from build123d import *

# Parameters (mm, degrees)
SKETCH1_R           = 34.671
BOSS_EXTRUDE1_DEPTH = 19.05
SKETCH5_R           = 5.08
CUT_EXTRUDE1_DEPTH  = 53.602841957
CHAMFER1_SIZE       = 6
CIRPATTERN1_COUNT   = 4
SKETCH8_R           = 3.3655
CUT_EXTRUDE2_DEPTH  = 53.602841957
CIRPATTERN2_COUNT   = 6


with BuildPart() as part:
    # Sketch1 → Boss-Extrude1 (new body)
    with BuildSketch(Plane(origin=(0, 0, 0), x_dir=(1, 0, 0), z_dir=(0, 1, 0))):
        with Locations(Location((0, 0, 0), (0, 0, 90))):
            Circle(SKETCH1_R)
    extrude(amount=BOSS_EXTRUDE1_DEPTH)

    # Sketch5 → Cut-Extrude1 (cut, through all)
    with BuildSketch(Plane.XZ):
        with Locations(Location((0, 0, 0), (0, 0, 270))):
            Circle(SKETCH5_R)
    extrude(amount=-CUT_EXTRUDE1_DEPTH, mode=Mode.SUBTRACT)

    # Chamfer1
    chamfer1_edges = [part.edges().sort_by_distance(p)[0] for p in [
        (0, 19.05, 5.08),
    ]]
    chamfer(chamfer1_edges, length=CHAMFER1_SIZE)

    # Sketch6 → #6-32 Tapped Hole1 (revolve, cut)
    with BuildSketch(Plane(origin=(0, 19.05, -13.5), x_dir=(0, 0, 1), z_dir=(1, 0, 0))):
        Polygon((0, 0), (0, 10.81269403), (1.35255, 10), (1.35255, 0), align=None)
    f_6_32_tapped_hole1 = revolve(axis=Axis((0, 25.4, -13.5), (0, -1, 0)), mode=Mode.SUBTRACT)

    # CirPattern1: #6-32 Tapped Hole1 ×4 about axis
    cirpattern1_axis = Axis((0, 0, 0), (0, 1, 0))
    for i in range(1, CIRPATTERN1_COUNT):
        add(f_6_32_tapped_hole1.rotate(cirpattern1_axis, i * 360 / CIRPATTERN1_COUNT), mode=Mode.SUBTRACT)

    # Sketch8 → Cut-Extrude2 (cut, through all)
    with BuildSketch(Plane(origin=(0, 19.05, 0), x_dir=(1, 0, 0), z_dir=(0, 1, 0))):
        with Locations(Location((0, 29.3624, 0), (0, 0, 270))):
            Circle(SKETCH8_R)
    cut_extrude2 = extrude(amount=-CUT_EXTRUDE2_DEPTH, mode=Mode.SUBTRACT)

    # CirPattern2: Cut-Extrude2 ×6 about axis
    cirpattern2_axis = Axis((0, 0, 0), (0, 1, 0))
    for i in range(1, CIRPATTERN2_COUNT):
        add(cut_extrude2.rotate(cirpattern2_axis, i * 360 / CIRPATTERN2_COUNT), mode=Mode.SUBTRACT)

    # Sketch9 → Cut-Revolve1 (revolve, cut)
    with BuildSketch(Plane.XY, mode=Mode.PRIVATE) as cut_revolve1_sk:
        Polygon((0, -2.570803014), (0, 0.5), (22.5, 0.5), (22.5, 0), (24.5, 0.5), (24.5, -7.98797561), (0, -7.98797561), align=None)
    cut_revolve1 = revolve(cut_revolve1_sk.sketch.rotate(Axis((0, -2.570803014, 0), (0, 1, 0)), 90), axis=Axis((0, -2.570803014, 0), (0, 1, 0)), mode=Mode.SUBTRACT)

    # Mirror1: Cut-Revolve1 across plane
    add(cut_revolve1.mirror(Plane(origin=(0, 9.525, 0), x_dir=(0, 0, 1), z_dir=(0, -1, 0))), mode=Mode.SUBTRACT)


solid = part.part
The model under review builds one solid part; all positions refer to its coordinate system, in mm. A direction names the side the tool comes from. Round coordinates to 2 decimals unless told otherwise and drop trailing zeros. Write each loop counter-clockwise with the first axis right and the second up, starting at its lowest first coordinate (ties: lowest second). Pieces come first, ordered by that corner, then holes. Notation, with made-up numbers: M -8,47 L 32,47 A3 ccw 32,51 Z; hole C 60.5,32 d10. An arc over 180 degrees is marked long. Answer as CSV lines item,"result". Start each with the question number.
Q1. Tool access review of faces 4 (the face through (-5.3, 0.5, -0.3)), 5 (the face through (10, 18.55, 5)), 6 (the face through (-23, 0, 10)): name each direction out of +Z, -Z, +X, -X, +Y, -Y from which nothing blocks a thin tool from reaching the whole face with its end or side.
Q2. Consider section B-B, the plane x = -26.5. Give the boundary of the cut face in (y, z), then the cut area to 3 significant figures.
Q3. Consider section A-A, the plane z = -29. Give the boundary of the cut face in (x, y).
Q4. Wall thickness on line 1 along Z through (x, y) = (26.5, 4); line 2 along X through (y, z) = (14, 13.5); line 3 along Y through (x, z) = (2.5, 13.5): over which ranges is each line inside the solid? List them lowest first.
Q5. Consider section D-D, the plane y = 16. State how many separate pieces and enclosed holes the cut face has, then the cut area to 3 significant figures.
Q6. The part is to be moulded in two halves that separate along Z. For faces 1 (the face through (-1.524, 9.392, 34.637)), 2 (the face through (-23, 19.05, 10)), 3 (the face through (0.148, 9.658, -32.725)), say which applies: +Z half, -Z half, draft (parallel to the pull), parting line (faces both ways), or undercut.
Q7. Clearance check with flat-ended pins moving along their axes: P1, Ø10, axis at y = 4, z = -17.5, coming from the -X side; P2, Ø10, axis at y = 7, z = -5.5, coming from the +X side; P3, Ø4, axis at x = 5, y = 5, coming from the -Z side. State where each tip first meets the part, or that it passes through.
Q8. Consider section C-C, the plane y = 5. Give the boundary of the cut face in (x, z), then the cut area to 3 significant figures.
Result set:
1,face 4,"-Y"
1,face 5,"+Y"
1,face 6,"+Z, -Z, +X, -X, -Y"
2,outline,"M 0,-22.36 L 19.05,-22.36 L 19.05,-17.87 L 0,-17.87 Z; M 0,-11.49 L 19.05,-11.49 L 19.05,11.49 L 0,11.49 Z; M 0,17.87 L 19.05,17.87 L 19.05,22.36 L 0,22.36 Z"
2,area,"609 mm²"
3,outline,"M -19,0 L -3.35,0 L -3.35,19.05 L -19,19.05 Z; M 3.35,0 L 19,0 L 19,19.05 L 3.35,19.05 Z"
4,line 1,"z = -22.36 to -17.87, -11.49 to 11.49, 17.87 to 22.36"
4,line 2,"x = -31.93 to -28.58, -22.28 to -1.35, 1.35 to 22.28, 28.58 to 31.93"
4,line 3,"y = 0.5 to 18.55"
5,separate pieces,"1"
5,enclosed holes,"11"
5,area,"3,340 mm²"
6,face 1,"parting line"
6,face 2,"draft"
6,face 3,"undercut"
7,P1,"stops at x = -32.34"
7,P2,"stops at x = 34.67"
7,P3,"stops at z = -34.54"
8,outline,"C 0,0 d69.34; hole C -25.43,-14.68 d6.73; hole C -25.43,14.68 d6.73; hole C 0,0 d10.16; hole C 0,-29.36 d6.73; hole C 0,29.36 d6.73; hole C 25.43,-14.68 d6.73; hole C 25.43,14.68 d6.73"
8,area,"3,480 mm²"
